Check sheet for the modelled part. Datum: model origin and axes. Units: mm. A direction names the side the tool comes from. Give positions to 0.01 mm unless a question says otherwise; leave off trailing zeros. Loops run counter-clockwise (first coordinate to the right, second up) from the corner with the lowest first, then second, coordinate; pieces in that order, holes last. Notation, with made-up numbers: M 58,64.25 L 81,64.25 A31 cw 81,96.25 Z; hole C 66.25,-37.5 d8. An arc over 180 degrees is marked long. Put each result on its own line as item: value. Start each with the question number.
```python
from build123d import *

# Parameters (mm, degrees)
F0_W     = 63.5
F0_H     = 116.84
F1_DEPTH = 12.7
F2_W     = 116.84
F2_H     = 7.6035529703
F2_R     = 1.7093941464
F3_DEPTH = 2.54


with BuildPart() as f1:
    # F0 (on Top) → F1 (new body)
    with BuildSketch(Plane.XY):
        Rectangle(F0_W, F0_H)
    extrude(amount=F1_DEPTH)

    # F2 (on face) → F3 (join)
    with BuildSketch(Plane(origin=(-31.75, 0, 0), x_dir=(0, -1, 0), z_dir=(-1, 0, 0))):
        with Locations((0, 16.5017764851)):
            Rectangle(F2_W, F2_H)
        with Locations((-50.292, 16.51)):
            Circle(F2_R, mode=Mode.SUBTRACT)
        with Locations((-35.3977816476, 16.51)):
            Circle(F2_R, mode=Mode.SUBTRACT)
        with Locations((-20.5035632952, 16.51)):
            Circle(F2_R, mode=Mode.SUBTRACT)
        with Locations((-5.6093449428, 16.51)):
            Circle(F2_R, mode=Mode.SUBTRACT)
        with Locations((9.2848734097, 16.51)):
            Circle(F2_R, mode=Mode.SUBTRACT)
        with Locations((24.1790917621, 16.51)):
            Circle(F2_R, mode=Mode.SUBTRACT)
    extrude(amount=-F3_DEPTH)


solid = f1.part
```
Q1. Section check C-C, the plane x = 5. Record the cut outline in (y, z).
Q2. Depth check by flat-ended pin: P1, Ø8, axis at x = -7.5, y = 12, coming from the +Z side; P2, Ø6, axis at y = -27.5, z = 16.5, coming from the +X side. Enter the tip coordinate at first touch or a pass-through.
Q3. Access from +Z, -Z, +X, -X, +Y, -Y to the whole of each face (thin tool, end or side, straight path). Record for faces 5 (the face through (1, 1, 12.7)), 6 (the face through (-30.498, 35.62, 18.205)).
Q4. Section check D-D, the plane y = -18.5. Record the cut outline in (x, z).
Q5. Section check B-B, the plane y = 6. Record the cut outline in (x, z).
Q6. Thickness scan on line 1 along Z through (x, y) = (-15.5, 15); line 2 along X through (y, z) = (52, 15.5). Record the ranges inside material, lowest first. Write a range as [from, to].
Q7. Section check A-A, the plane z = 16.51. Record the cut outline in (x, y), then the cut area to 3 significant figures.
Q8. Mould release check, pull along Z, two halves, no side actions. Record for faces 1 (the face through (-29.21, 1, 17)), 2 (the face through (-30, 1, 20.304)), 3 (the face through (-30.498, 5.832, 18.205)), 4 (the face through (-30.5, 52, 16.6)): pulls with the +Z half, pulls with the -Z half, needs draft (parallel to the pull), parting line crosses it, or undercut.
Found:
1. outline: M -58.42,0 L 58.42,0 L 58.42,12.7 L -58.42,12.7 Z
2. P1: stops at z = 12.7
2. P2: stops at x = -29.21
3. face 5: +Z, +X, +Y, -Y
3. face 6: +X, -X
4. outline: M -31.75,0 L 31.75,0 L 31.75,12.7 L -29.21,12.7 L -29.21,20.3 L -31.75,20.3 Z
5. outline: M -31.75,0 L 31.75,0 L 31.75,12.7 L -29.21,12.7 L -29.21,14.85 L -31.75,14.85 Z; M -31.75,18.17 L -29.21,18.17 L -29.21,20.3 L -31.75,20.3 Z
6. line 1: z = [0, 12.7]
6. line 2: x = [-31.75, -29.21]
7. outline: M -31.75,-58.42 L -29.21,-58.42 L -29.21,-25.89 L -31.75,-25.89 Z; M -31.75,-22.47 L -29.21,-22.47 L -29.21,-10.99 L -31.75,-10.99 Z; M -31.75,-7.58 L -29.21,-7.58 L -29.21,3.9 L -31.75,3.9 Z; M -31.75,7.32 L -29.21,7.32 L -29.21,18.79 L -31.75,18.79 Z; M -31.75,22.21 L -29.21,22.21 L -29.21,33.69 L -31.75,33.69 Z; M -31.75,37.11 L -29.21,37.11 L -29.21,48.58 L -31.75,48.58 Z; M -31.75,52 L -29.21,52 L -29.21,58.42 L -31.75,58.42 Z
7. area: 245 mm^2
8. face 1: needs draft
8. face 2: pulls with the +Z half
8. face 3: undercut
8. face 4: undercut
